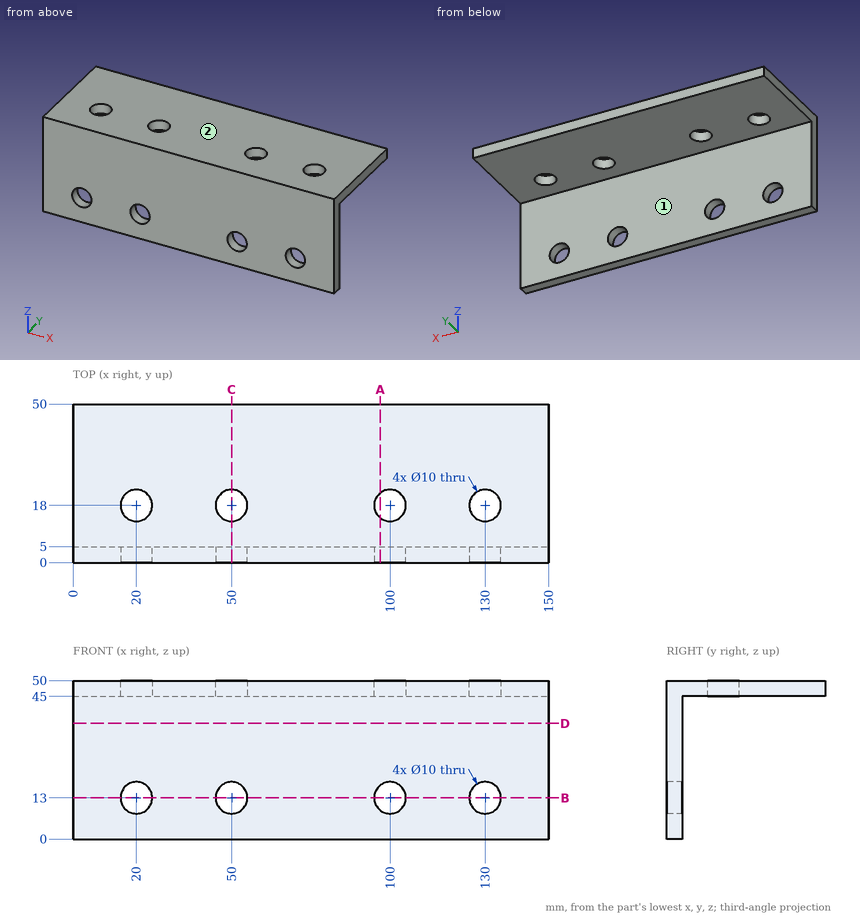
Could you check a few things on this drawing? It's one solid part, dimensions in mm from its lowest x, y, z. A direction names the side the tool comes from. Coordinates: 2 decimals unless noted, no trailing zeros. Write each loop counter-clockwise with the first axis right and the second up, starting at its lowest first coordinate (ties: lowest second). Pieces come first, ordered by that corner, then holes. Notation, with made-up numbers: (46.5, -29.75) - (93.5, -29.75) arc R23 cw to (93.5, -8.75) - close; hole circle Ø4 at (-4, 71.25). An arc over 180 degrees is marked (long way). Return JSON: item names as keys, results as strings. Group by question number.
Item 1: I'm going to push flat-ended pins straight in: pin 1 Ø13.5 at (x, z) = (61.5, 27.5) entering from +Y; pin 2 Ø9 at (x, y) = (50, 18) entering from -Z; pin 3 Ø1 at (x, y) = (32, 45) entering from -Z. Where does each tip first touch, or does it pass through?
Item 2: If we section it at B-B (z = 13): Write out the boundary of the cut face in (x, y), then the cut area to 3 significant figures.
Item 3: If we section it at D-D (z = 36.5): Write out the boundary of the cut face in (x, y), then the cut area to 3 significant figures.
Item 4: Which directions (+Z, -Z, +X, -X, +Y, -Y) give clear straight access to the entire face, cutting with the end or side of a thin tool? Please do the marked faces 1 and 2.
Item 5: If we section it at A-A (x = 97): Write out the boundary of the cut face in (y, z).
Item 6: Please list where these lines run through material, in increasing order: probe 1 along Y at (x, z) = (50, 48.7); probe 2 along Y at (x, z) = (81, 4); probe 3 along Z at (x, y) = (136, 46).
Item 7: If we section it at C-C (x = 50): Write out the boundary of the cut face in (y, z).
Return value:
{
 "1": {"pin 1": "stops at y = 5", "pin 2": "passes through", "pin 3": "stops at z = 45"},
 "2": {"outline": "(0, 0) - (15, 0) - (15, 5) - (0, 5) - close; (25, 0) - (45, 0) - (45, 5) - (25, 5) - close; (55, 0) - (95, 0) - (95, 5) - (55, 5) - close; (105, 0) - (125, 0) - (125, 5) - (105, 5) - close; (135, 0) - (150, 0) - (150, 5) - (135, 5) - close", "area": "550 mm^2"},
 "3": {"outline": "(0, 0) - (150, 0) - (150, 5) - (0, 5) - close", "area": "750 mm^2"},
 "4": {"face 1": "-Z, +X, -X, +Y", "face 2": "+Z, +X, -X, +Y, -Y"},
 "5": {"outline": "(0, 0) - (5, 0) - (5, 9) - (0, 9) - close; (0, 17) - (5, 17) - (5, 45) - (14, 45) - (14, 50) - (0, 50) - close; (22, 45) - (50, 45) - (50, 50) - (22, 50) - close"},
 "6": {"probe 1": "y = 0 to 13, 23 to 50", "probe 2": "y = 0 to 5", "probe 3": "z = 45 to 50"},
 "7": {"outline": "(0, 0) - (5, 0) - (5, 8) - (0, 8) - close; (0, 18) - (5, 18) - (5, 45) - (13, 45) - (13, 50) - (0, 50) - close; (23, 45) - (50, 45) - (50, 50) - (23, 50) - close"}
}
